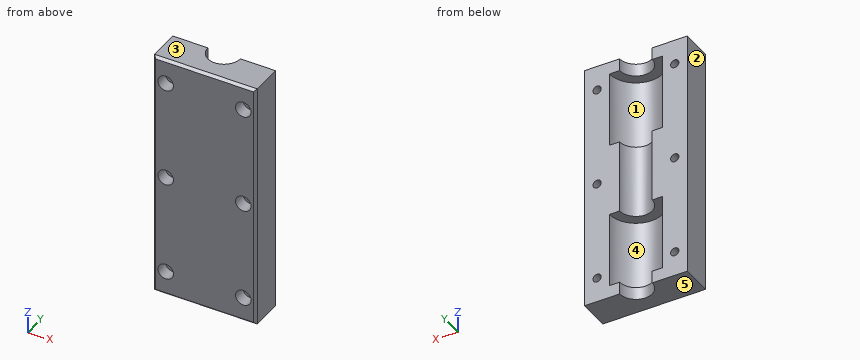
```python
from build123d import *

# Parameters (mm, degrees)
PAD_DEPTH       = 50
SKETCH001_R     = 1.65
POCKET_DEPTH    = 13.501
SKETCH002_R     = 3.1
POCKET001_DEPTH = 5
SKETCH003_R     = 10.6
POCKET002_DEPTH = 30.3
SKETCH004_R     = 10.6
POCKET003_DEPTH = 30.3
CHAMFER_SIZE    = 1


with BuildPart() as part:
    # Sketch → Pad (new body, symmetric)
    with BuildSketch(Plane.XY):
        with BuildLine():
            Line((-20.5, -13.5), (20.5, -13.5))
            Line((20.5, -13.5), (20.5, 0))
            Line((20.5, 0), (6.5, 0))
            ThreePointArc((-6.5, 0), (0, -6.5), (6.5, 0))
            Line((-6.5, 0), (-20.5, 0))
            Line((-20.5, 0), (-20.5, -13.5))
        make_face()
    extrude(amount=PAD_DEPTH, both=True)

    # Sketch001 → Pocket (cut, through all)
    with BuildSketch(Plane.XZ):
        with Locations((-15.5, 40)):
            Circle(SKETCH001_R)
        with Locations((-15.5, 0)):
            Circle(SKETCH001_R)
        with Locations((-15.5, -40)):
            Circle(SKETCH001_R)
        with Locations((15.5, -40)):
            Circle(SKETCH001_R)
        with Locations((15.5, 0)):
            Circle(SKETCH001_R)
        with Locations((15.5, 40)):
            Circle(SKETCH001_R)
    extrude(amount=POCKET_DEPTH, mode=Mode.SUBTRACT)

    # Sketch002 (on Face1 of Pocket) → Pocket001 (cut)
    with BuildSketch(Plane.XZ.offset(13.5)):
        with Locations((-15.5, 40)):
            Circle(SKETCH002_R)
        with Locations((15.5, 40)):
            Circle(SKETCH002_R)
        with Locations((15.5, 0)):
            Circle(SKETCH002_R)
        with Locations((-15.5, 0)):
            Circle(SKETCH002_R)
        with Locations((-15.5, -40)):
            Circle(SKETCH002_R)
        with Locations((15.5, -40)):
            Circle(SKETCH002_R)
    extrude(amount=-POCKET001_DEPTH, mode=Mode.SUBTRACT)

    # Sketch003 (on DatumPlane) → Pocket002 (cut)
    with BuildSketch(Plane.XY.offset(45)):
        Circle(SKETCH003_R)
    extrude(amount=-POCKET002_DEPTH, mode=Mode.SUBTRACT)

    # Sketch004 (on DatumPlane) → Pocket003 (cut)
    with BuildSketch(Plane.XY.offset(-45)):
        Circle(SKETCH004_R)
    extrude(amount=POCKET003_DEPTH, mode=Mode.SUBTRACT)

    # Chamfer
    chamfer_edges = [part.edges().sort_by_distance(p)[0] for p in [
        (20.5, -13.5, 0),
        (0, -13.5, 50),
        (-20.5, -13.5, 0),
        (0, -13.5, -50),
    ]]
    chamfer(chamfer_edges, length=CHAMFER_SIZE)


solid = part.part
```
Read the model definition and answer for the solid it produces. Units are mm, in the model's axes. Face numbers are marked on the shaded views. A direction names the side the tool comes from. Round coordinates to 2 decimals unless told otherwise and drop trailing zeros. Write each loop counter-clockwise with the first axis right and the second up, starting at its lowest first coordinate (ties: lowest second). Pieces come first, ordered by that corner, then holes. Notation, with made-up numbers: (58, 53) - (92, 53) arc R12 cw to (92, 68) - close; hole circle Ø2 at (-17.75, 57). An arc over 180 degrees is marked (long way). One line per item, written item: value.
Q1. Straight lines are drawn through the part: line 1 (Z direction, x = 10, y = -2); line 2 (Z direction, x = 15.5, y = -11.6); line 3 (Z direction, x = 15.5, y = -6). For each, find the intervals that lie inside material, in ascending order. Write a range as from..to.
The answers:
line 1: z = -50..-45, -14.7..14.7, 45..50
line 2: z = -50..-43.1, -36.9..-3.1, 3.1..36.9, 43.1..50
line 3: z = -50..-41.65, -38.35..-1.65, 1.65..38.35, 41.65..50
Q2. Find section B-B (y = -1). Count the separate pieces of the cut face and the enclosed holes in it, and give its area (3 significant figures).
The answers:
separate pieces: 2
enclosed holes: 6
area: 2,260 mm2
Q3. Find section D-D (z = -12). Determine the outline of the cut face in (x, y).
The answers:
outline: (-20.5, -12.5) - (-19.5, -13.5) - (19.5, -13.5) - (20.5, -12.5) - (20.5, 0) - (6.5, 0) arc R6.5 cw to (-6.5, 0) - (-20.5, 0) - close
Q4. Find section C-C (x = 0). Determine the outline of the cut face in (y, z).
The answers:
outline: (-13.5, -49) - (-12.5, -50) - (-6.5, -50) - (-6.5, -45) - (-10.6, -45) - (-10.6, -14.7) - (-6.5, -14.7) - (-6.5, 14.7) - (-10.6, 14.7) - (-10.6, 45) - (-6.5, 45) - (-6.5, 50) - (-12.5, 50) - (-13.5, 49) - close
Q5. Each of these flat-tipped pins is pushed along its axis until it touches: P1, Ø3.5, axis at x = -15.5, z = 40, coming from the -Y side; P2, Ø2, axis at x = -15.5, z = 40, coming from the -Y side (3 decimals); P3, Ø10, axis at x = -15.5, z = -40, coming from the -Y side. Where does it stop, or does it pass through?
The answers:
P1: stops at y = -8.5
P2: passes through
P3: stops at y = -13.5
Q6. Which of the six approach directions +Z, -Z, +X, -X, +Y, -Y give full straight-line access (tool end or side, diameter ignored) to the marked faces 4 and 5?
The answers:
face 4: +Y
face 5: -Z, +X, -X, +Y, -Y
Q7. Find section A-A (z = -40). Determine the outline of the cut face in (x, y).
The answers:
outline: (-20.5, -12.5) - (-19.5, -13.5) - (-18.6, -13.5) - (-18.6, -8.5) - (-17.15, -8.5) - (-17.15, 0) - (-20.5, 0) - close; (-13.85, -8.5) - (-12.4, -8.5) - (-12.4, -13.5) - (12.4, -13.5) - (12.4, -8.5) - (13.85, -8.5) - (13.85, 0) - (10.6, 0) arc R10.6 cw to (-10.6, 0) - (-13.85, 0) - close; (17.15, -8.5) - (18.6, -8.5) - (18.6, -13.5) - (19.5, -13.5) - (20.5, -12.5) - (20.5, 0) - (17.15, 0) - close
Q8. For a pull along X with two mould halves and no side action, classify the marked faces 1, 2 and 3 as pulls with the +X half, pulls with the -X half, needs draft (parallel to the pull), parting line crosses it, or undercut.
The answers:
face 1: undercut
face 2: pulls with the -X half
face 3: needs draft
